For this review, take the finished solid that the model builds, in its own axes (mm). Face numbers are marked on the shaded views. A direction names the side the tool comes from. Coordinates: 2 decimals unless noted, no trailing zeros. Loops run counter-clockwise (first coordinate to the right, second up) from the corner with the lowest first, then second, coordinate; pieces in that order, holes last. Notation, with made-up numbers: M -30.5,-25 L 3.5,-25 A30 ccw 3.5,-3 Z; hole C -23,-14 d1. An arc over 180 degrees is marked long. Answer as a JSON object with one key per item and string values. Group by question number.
Item 1: Add section C-C (z = 44.5). State the section outline as (x, y) points.
Item 2: Tool access review of the marked faces 1 and 2: name each direction out of +Z, -Z, +X, -X, +Y, -Y from which nothing blocks a thin tool from reaching the whole face with its end or side.
Item 3: Add section D-D (z = 17.5). State the section outline as (x, y) points.
Item 4: Wall thickness on L1, parallel to Y at x = 0, z = 48.5; L2, parallel to Z at x = -5.75, y = 2.25; L3, parallel to Z at x = 0.5, y = 2.25: over which ranges is each line inside the solid? List them lowest first. Write a range as from..to.
Item 5: Add section B-B (x = 0.25). State the section outline as (y, z) points, then the cut area to 3 significant figures.
Item 6: Insertion check: pin 1 (6 mm diameter, centred on y = 2, z = 4.5, fed in from -X); pin 2 (1.5 mm diameter, centred on x = -1, y = 1, fed in from +Z); pin 3 (5 mm diameter, centred on y = -3, z = 35.5, fed in from +X). Each pin has a flat end and moves straight along its axis. Give the tip position at first contact, or say it passes through.
Item 7: Add section A-A (y = 0). State the section outline as (x, z) points.
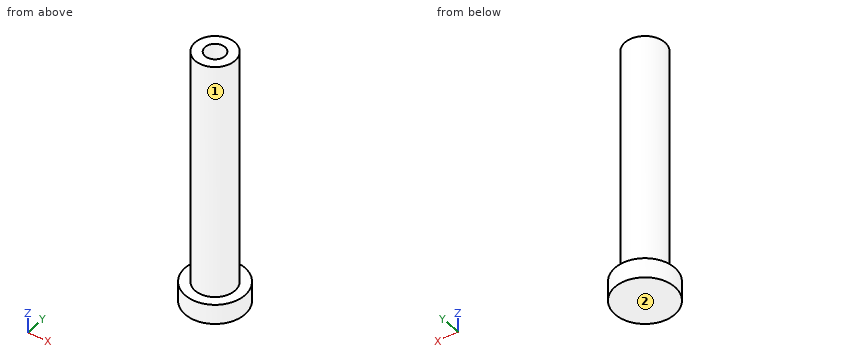
from build123d import *

# Parameters (mm, degrees)
F0_R     = 5
F1_DEPTH = 60
F2_R     = 7.5
F2_R_2   = 5
F3_DEPTH = 5
F4_R     = 2.5
F5_DEPTH = 25


with BuildPart() as f1:
    # F0 (on Top) → F1 (new body)
    with BuildSketch(Plane.XY):
        Circle(F0_R)
    extrude(amount=F1_DEPTH)

    # F2 (on face) → F3 (join)
    with BuildSketch(Plane(origin=(0, 0, 0), x_dir=(1, 0, 0), z_dir=(0, 0, -1))):
        Circle(F2_R)
        Circle(F2_R_2, mode=Mode.SUBTRACT)
        Circle(F2_R_2)
    extrude(amount=F3_DEPTH)

    # F4 (on face) → F5 (cut)
    with BuildSketch(Plane.XY.offset(60)):
        Circle(F4_R)
    extrude(amount=-F5_DEPTH, mode=Mode.SUBTRACT)


solid = f1.part
From the geometry:
{
 "1": {"outline": "C 0,0 d10; hole C 0,0 d5"},
 "2": {"face 1": "+Z", "face 2": "-Z, +X, -X, +Y, -Y"},
 "3": {"outline": "C 0,0 d10"},
 "4": {"L1": "y = -5..-2.5, 2.5..5", "L2": "z = -5..0", "L3": "z = -5..35"},
 "5": {"outline": "M -7.5,-5 L 7.5,-5 L 7.5,0 L 4.99,0 L 4.99,60 L 2.49,60 L 2.49,35 L -2.49,35 L -2.49,60 L -4.99,60 L -4.99,0 L -7.5,0 Z", "area": "550 mm²"},
 "6": {"pin 1": "stops at x = -5", "pin 2": "stops at z = 35", "pin 3": "stops at x = 4.97"},
 "7": {"outline": "M -7.5,-5 L 7.5,-5 L 7.5,0 L 5,0 L 5,60 L 2.5,60 L 2.5,35 L -2.5,35 L -2.5,60 L -5,60 L -5,0 L -7.5,0 Z"}
}
